Part model, mm, in its own coordinate system. A direction names the side the tool comes from. Coordinates: 2 decimals unless noted, no trailing zeros.
1) Wall check: L1, parallel to Z at x = 8, y = 1.2 (1 decimal); L2, parallel to Z at x = 8, y = 2.9 (1 decimal); L3, parallel to Z at x = -20, y = 1 (3 decimals). Give the ranges that are in metal, low to high.
2) Mould opens along X. For faces 3 (the cylindrical face through (8.992, 3.24, -12.686)), 4 (the flat face through (-2, 4, -7)), 5 (the cylindrical face through (-5.347, 1.626, -10.939)) say: +X half, -X half, draft (parallel to the pull), parting line (faces both ways), or undercut.
3) Pin check, flat tips, straight feed: pin 1 Ø1.5 at (x, z) = (8, -22.97) entering from -Y; pin 2 Ø3 at (x, z) = (8, -13.45) entering from -Y. Stop position of each tip, or through.
4) Cut at A-A (y = 0.65). Give the number of separate pieces and of enclosed holes in the cut face, and give its area (3 significant figures).
5) Tool access for faces 1 (the flat face through (8, 2.5, -15)), 2 (the cylindrical face through (-21.89, 1.63, -5.49)): list every direction of +Z, -Z, +X, -X, +Y, -Y with a clear straight run to the whole face (end or side of a thin tool).
Autodesk Inventor part; units mm, degrees
ref_plane "YZ Plane" through (0, 0, 0) normal (1, 0, 0) x (0, 1, 0)
ref_plane "XZ Plane" through (0, 0, 0) normal (0, 1, 0) x (-1, 0, 0)
ref_plane "XY Plane" through (0, 0, 0) normal (0, 0, 1) x (1, 0, 0)
sketch "Sketch1" plane through (0, 0, 0) normal (0, 1, 0) x (-1, 0, 0)
  circle A0 centre (0, 0) radius 2.63
  circle A1 centre (20, 0) radius 2.63
  circle A2 centre (-8, -13.4465) radius 1.25
  circle A3 centre (-8, -22.9715) radius 1.25
  circle A4 centre (20, 0) radius 5.805 construction
  circle A5 centre (0, 0) radius 5.805 construction
  circle A6 centre (-8, -13.4465) radius 4.425 construction
  circle A7 centre (-8, -22.9715) radius 4.425 construction
  line L0 (20, 5.805) -> (-9.25, 5.805)
  line L1 (-12.425, 2.63) -> (-12.425, -22.9715)
  line L2 (23.5083, -4.625) -> (-5.3257, -26.497)
  arc A8 (23.5083, -4.625) -> (20, 5.805) centre (20, 0) ccw
  arc A9 (-12.425, -22.9715) -> (-5.3257, -26.497) centre (-8, -22.9715) ccw
  arc A10 (-9.25, 5.805) -> (-12.425, 2.63) centre (-9.25, 2.63) ccw
  point P0 (0, 10)
  dimension "d0" = 5.26
  dimension "d1" = 20
  dimension "d2" = 2.5
  dimension "d3" = 10
  dimension "d4" = 13.4465
  dimension "d5" = 8
  dimension "d6" = 9.525
  dimension "d7" = 3.175
  dimension "d8" = 3.175
  dimension "d9" = 3.175
extrude "Extrusion1" add sketch "Sketch1" along normal blind 4
sketch "Sketch2" plane through (0, 0, 0) normal (0, -1, 0) x (1, 0, 0)
  circle A0 centre (8, -13.4465) radius 1.25
  circle A1 centre (8, -22.9715) radius 1.25
  circle A2 centre (8, -13.4465) radius 2
  circle A3 centre (8, -22.9715) radius 2
  point P0 (0, 0)
  dimension "d12" = 4
extrude "Extrusion2" cut sketch "Sketch2" against normal blind 2.5
sketch "Sketch3" plane through (0, 4, 0) normal (0, 1, 0) x (1, 0, 0)
  circle A0 centre (-20, 0) radius 2.63
  circle A1 centre (8, 22.9715) radius 1.25
  circle A2 centre (-20, 0) radius 5.805 construction
  circle A3 centre (8, 22.9715) radius 4.425 construction
  arc A4 (-23.5083, 4.625) -> (-20, -5.805) centre (-20, 0) ccw
  arc A5 (12.425, 22.9715) -> (5.3257, 26.497) centre (8, 22.9715) ccw
  circle A6 centre (0, 0) radius 5.805 construction
  circle A7 centre (8, 13.4465) radius 1.25 construction
  circle A8 centre (8, 13.4465) radius 4.425 construction
  arc A9 (-20.1243, 5.8037) -> (3.7466, 24.192) centre (-20.6681, 31.1978) ccw
  arc A10 (-20.1243, 5.8037) -> (-23.5083, 4.625) centre (-20, 0) ccw
  arc A11 (5.3257, 26.497) -> (3.7466, 24.192) centre (8, 22.9715) ccw
  line L0 (5.3257, 26.497) -> (-23.5083, 4.625)
  dimension "d15" = 25.4
extrude "Extrusion3" cut sketch "Sketch3" against normal through all contours A10 L0 A11 A9
chamfer "Chamfer1" distance 0.7937 angle 45 6 edges at (12.425, 4, -10.1707) (8.6163, 4, -27.3534) (-5.1676, 4, -11.0758) (-25.8047, 4, 0.0621) (-5.375, 4, 5.805) (11.4951, 4, 4.8751)
properties part number "CNC-021-ZAxisLimitSwitchMount" material "ABS Plastic"
Geometry check:
1. L1: z = -27.4 to -25, -21 to -15.4, -11.4 to 5.8
1. L2: z = -27.4 to -24.2, -21.7 to -14.7, -12.2 to 5.8
1. L3: z = -5.807 to -2.63, 2.63 to 5.805
2. face 3: undercut
2. face 4: draft
2. face 5: -X half
3. pin 1: passes through
3. pin 2: stops at y = 2.5
4. separate pieces: 1
4. enclosed holes: 4
4. area: 656 mm2
5. face 1: -Y
5. face 2: -Z, -X, +Y, -Y
